```python
from build123d import *

# Parameters (mm, degrees)
CROQUIS1_R              = 4.446768191
SALIENTE_EXTRUIR1_DEPTH = 3


with BuildPart() as part:
    # Croquis1 → Saliente-Extruir1 (new body)
    with BuildSketch(Plane(origin=(0, 0, 0), x_dir=(1, 0, 0), z_dir=(0, 1, 0))):
        with BuildLine():
            ThreePointArc((0.04624071, -5.650316034), (5.650457939, 0.023120548), (0, 5.650505241))
            Line((0, 5.650505241), (-6.558714934, 5.650505241))
            Line((-6.558714934, 5.650505241), (-7.488201893, 5.650505241))
            ThreePointArc((-7.488201893, 5.650505241), (-7.823446184, 5.570700791), (-8.086776283, 5.348406518))
            ThreePointArc((-8.086776283, 5.348406518), (-10.345385807, 3.886616052), (-13.007001279, 4.2789825))
            ThreePointArc((-13.007001279, 4.2789825), (-16.387283849, 2.318589671), (-13.058926803, 0.271276879))
            ThreePointArc((-13.058926803, 0.271276879), (-12.757166646, 0.290746917), (-12.539738197, 0.080596626))
            ThreePointArc((-12.539738197, 0.080596626), (-13.014703567, -1.709451511), (-14.866296536, -1.747764912))
            ThreePointArc((-14.866296536, -1.747764912), (-15.955750761, -1.665010286), (-16.52578224, -2.597117012))
            ThreePointArc((-16.52578224, -2.597117012), (-16.279366787, -4.255127031), (-15.561421483, -5.769812589))
            ThreePointArc((-15.561421483, -5.769812589), (-13.964054479, -11.235683534), (-15.795045548, -16.627788712))
            ThreePointArc((-15.795045548, -16.627788712), (-16.170307553, -18.987627294), (-14.467414276, -20.663877332))
            ThreePointArc((-14.467414276, -20.663877332), (-13.433418752, -21.52247795), (-13.304756207, -22.860307429))
            ThreePointArc((-13.304756207, -22.860307429), (-15.728318678, -33.985404535), (-16.335024288, -45.355248377))
            ThreePointArc((-16.335024288, -45.355248377), (-15.195125313, -48.044049913), (-12.531403036, -49.241383204))
            ThreePointArc((-12.531403036, -49.241383204), (-11.635581739, -48.920558505), (-11.228904984, -48.060303717))
            ThreePointArc((-11.228904984, -48.060303717), (-8.826265832, -27.920860577), (-3.642833223, -8.31214131))
            ThreePointArc((-3.642833223, -8.31214131), (-2.222317675, -6.393569379), (0.04624071, -5.650316034))
        make_face()
        Circle(CROQUIS1_R, mode=Mode.SUBTRACT)
    extrude(amount=SALIENTE_EXTRUIR1_DEPTH)


solid = part.part
```
Build history of the part. All positions in model axes, mm. A direction names the side the tool comes from. Give positions to 0.01 mm unless a question says otherwise; leave off trailing zeros. Loops run counter-clockwise (first coordinate to the right, second up) from the corner with the lowest first, then second, coordinate; pieces in that order, holes last. Notation, with made-up numbers: (60, 28.25) - (78, 28.25) arc R31 ccw to (78, 60.25) - close; hole circle Ø4 at (41, -21). An arc over 180 degrees is marked (long way). Use a Markdown table: item, result.
(1) Drop a flat-ended pin along its axis: pin 1 Ø7 at (x, z) = (0, 0) entering from +Y. Give the stop position or say it passes through.
Taken from the geometry:
| item | result |
|---|---|
| pin 1 | through |
(2) Wall check: line 1 along Z through (x, y) = (-0.75, 1.25); line 2 along X through (y, z) = (1.25, 3); line 3 along Z through (x, y) = (-13, 1.1). Give the ranges that are in metal, low to high.
Taken from the geometry:
| item | result |
|---|---|
| line 1 | -5.65 to -4.38, 4.38 to 5.74 |
| line 2 | -16.51 to -3.28, 3.28 to 4.79 |
| line 3 | -4.28 to -0.3, 1.7 to 49.19 |
(3) Pull direction Z, two halves, no side cores. Call faces 3 (the face through (-13.44, 1.48, 21.51)), 4 (the face through (-15.941, 1.479, 1.658)), 5 (the face through (-2.25, 1.479, 6.414)), 6 (the face through (-10.308, 1.479, -3.895)): +Z half, -Z half, draft (parallel to the pull), parting line (faces both ways), or undercut.
Taken from the geometry:
| item | result |
|---|---|
| face 3 | undercut |
| face 4 | undercut |
| face 5 | +Z half |
| face 6 | -Z half |
(4) Which spindle directions (+Z, -Z, +X, -X, +Y, -Y) get a long thin tool onto all of the face, cutting with end or side? Do faces 1 (the face through (-15.707, 1.479, 33.827)), 2 (the face through (-11, 3, 15)). Say none if no direction does.
Taken from the geometry:
| item | result |
|---|---|
| face 1 | -X, +Y, -Y |
| face 2 | +Z, -Z, +X, -X, +Y |
(5) Band-saw the part on C-C (x = 2.5). Give the cut face in (y, z).
Taken from the geometry:
| item | result |
|---|---|
| outline | (0, -5.07) - (3, -5.07) - (3, -3.68) - (0, -3.68) - close; (0, 3.68) - (3, 3.68) - (3, 5.07) - (0, 5.07) - close |
(6) Band-saw the part on A-A (x = -1.5). Give the cut face in (y, z), and give its area (3 significant figures).
Taken from the geometry:
| item | result |
|---|---|
| outline | (0, -5.65) - (3, -5.65) - (3, -4.19) - (0, -4.19) - close; (0, 4.19) - (3, 4.19) - (3, 5.98) - (0, 5.98) - close |
| area | 9.78 mm2 |
(7) Band-saw the part on B-B (y = 2.1). Give the cut face in (x, z), and give its area (3 significant figures).
Taken from the geometry:
| item | result |
|---|---|
| outline | (-16.53, 2.6) arc R1.05 ccw to (-14.87, 1.75) arc R1.54 cw to (-12.54, -0.08) arc R0.37 cw to (-13.06, -0.27) arc R2.28 ccw (long way) to (-13.01, -4.28) arc R3.81 cw to (-8.09, -5.35) arc R0.74 ccw to (-7.49, -5.65) - (0, -5.65) arc R5.65 ccw to (0.05, 5.65) arc R3.93 cw to (-3.64, 8.31) arc R145.31 cw to (-11.23, 48.06) arc R1.24 ccw to (-12.53, 49.24) arc R4 ccw to (-16.34, 45.36) arc R70.72 ccw to (-13.3, 22.86) arc R1.76 cw to (-14.47, 20.66) arc R2.61 ccw to (-15.8, 16.63) arc R9.46 cw to (-15.56, 5.77) arc R5.7 ccw to start; hole circle Ø8.89 at (0, 0) |
| area | 459 mm2 |
(8) Band-saw the part on D-D (z = 6.5). Give the cut face in (x, y).
Taken from the geometry:
| item | result |
|---|---|
| outline | (-15.12, 0) - (-2.36, 0) - (-2.36, 3) - (-15.12, 3) - close |
